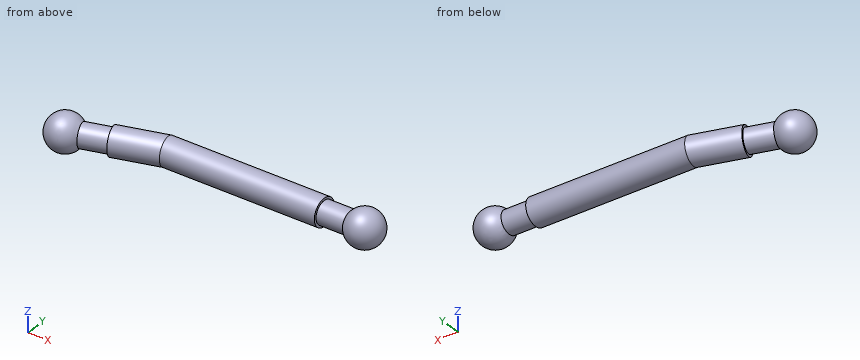
from build123d import *

# Parameters (mm, degrees)
SKETCH1_R           = 3
SKETCH3_R           = 2.5
BOSS_EXTRUDE1_DEPTH = 6
SKETCH5_R           = 2.5
BOSS_EXTRUDE2_DEPTH = 6


with BuildPart() as part:
    # Sweep2: sweep along a path in Sketch2
    with BuildLine(Plane.XY) as sweep2_path:
        Line((0, 0), (-35, 0))
        Line((-35, 0), (-45, -3))
    # Sketch1 → Sweep2 (sweep)
    with BuildSketch(Plane(origin=(0, 0, 0), x_dir=(0, 0, -1), z_dir=(1, 0, 0))):
        Circle(SKETCH1_R)
    sweep(path=sweep2_path.line, transition=Transition.RIGHT)

    # Sketch3 → Boss-Extrude1 (add)
    with BuildSketch(Plane(origin=(-42.110091743, -12.633027523, 0), x_dir=(0, 0, 1), z_dir=(-0.9578262852211515, -0.2873478855663453, 0))):
        with Locations(Location((0, 10.057175995, 0), (0, 0, 270))):
            Circle(SKETCH3_R)
    extrude(amount=BOSS_EXTRUDE1_DEPTH)

    # Sketch4 → Revolve1 (revolve)
    with BuildSketch(Plane(origin=(-50.73052831, -15.219158493, 0), x_dir=(0, 0, 1), z_dir=(-0.9578262852211515, -0.28734788556634533, 0))):
        with BuildLine():
            Line((0, 14.057175995), (0, 6.057175995))
            ThreePointArc((0, 6.057175995), (4, 10.057175995), (0, 14.057175995))
        make_face()
    revolve(axis=Axis((-54.769828109, -1.754825829, 0), (0.28734788556634544, -0.9578262852211514, 0)))

    # Sketch5 → Boss-Extrude2 (add)
    with BuildSketch(Plane(origin=(0, 0, 0), x_dir=(0, 0, -1), z_dir=(1, 0, 0))):
        Circle(SKETCH5_R)
    extrude(amount=BOSS_EXTRUDE2_DEPTH)

    # Sketch6 → Revolve2 (revolve)
    with BuildSketch(Plane(origin=(9, 0, 0), x_dir=(0, 0, -1), z_dir=(1, 0, 0))):
        with BuildLine():
            Line((0, 4), (0, -4))
            ThreePointArc((0, -4), (4, 0), (0, 4))
        make_face()
    revolve(axis=Axis((9, 4, 0), (0, -1, 0)))


solid = part.part
The model under review builds one solid part; all positions refer to its coordinate system, in mm. Round coordinates to 2 decimals unless told otherwise and drop trailing zeros. Write each loop counter-clockwise with the first axis right and the second up, starting at its lowest first coordinate (ties: lowest second). Pieces come first, ordered by that corner, then holes. Notation, with made-up numbers: M 5.25,6.5 L 30.25,6.5 A18 ccw 30.25,28.5 Z; hole C 43,89.25 d6. An arc over 180 degrees is marked long. Answer as CSV lines item,"result". Start each with the question number.
Q1. Wall thickness on line 1 along Z through (x, y) = (-29, 0); line 2 along X through (y, z) = (-6.75, 1.75); line 3 along X through (y, z) = (-7, -1): over which ranges is each line inside the solid? List them lowest first.
Q2. Clearance check with flat-ended pins moving along their axes: P1, Ø3, axis at y = -2, z = 2, coming from the +X side; P2, Ø4, axis at y = -0.5, z = 2.5, coming from the +X side; P3, Ø1, axis at x = -10.5, y = 0, coming from the +Z side. State where each tip first meets the part, or that it passes through.
Q3. Consider section A-A, the plane z = 0. Give the boundary of the cut face in (x, y), then the cut area to 3 significant figures.
Result set:
1,line 1,"z = -3 to 3"
1,line 2,"x = -57.02 to -50.22"
1,line 3,"x = -57.23 to -50.01"
2,P1,"stops at x = 12.77"
2,P2,"stops at x = 12.96"
2,P3,"stops at z = 3"
3,outline,"M -51.35,-2.29 A4 ccw long -49.91,-7.08 L -44.28,-5.39 L -44.14,-5.87 L -34.56,-3 L 0,-3 L 0,-2.5 L 5.88,-2.5 A4 ccw long 5.88,2.5 L 0,2.5 L 0,3 L -35.44,3 L -45.86,-0.13 L -45.72,-0.61 Z"
3,area,"426 mm²"
